For this review, take the finished solid that the model builds, in its own axes (mm). A direction names the side the tool comes from. Round coordinates to 2 decimals unless told otherwise and drop trailing zeros. Write each loop counter-clockwise with the first axis right and the second up, starting at its lowest first coordinate (ties: lowest second). Pieces come first, ordered by that corner, then holes. Notation, with made-up numbers: (83, 59.25) - (108, 59.25) arc R13 ccw to (108, 81.25) - close; hole circle Ø5 at (20.5, 19.25). An arc over 180 degrees is marked (long way). One line per item, written item: value. Start each with the question number.
Q1. Add section D-D on y = -4. Write out the cut boundary in (x, z), and give its area (3 significant figures).
Q2. Tool access review of faces 4 (the face through (-45, 1, 25.4)), 5 (the face through (-88.9, 13, 13)), 6 (the face through (38.1, -13, 38)), 7 (the face through (-64, -38.1, 13)): name each direction out of +Z, -Z, +X, -X, +Y, -Y from which nothing blocks a thin tool from reaching the whole face with its end or side.
Q3. Add section B-B on y = 22. Write out the cut boundary in (x, z), and give its area (3 significant figures).
Q4. Clearance check with flat-ended pins moving along their axes: pin 1 Ø20.5 at (x, z) = (-63.5, 15.5) entering from -Y; pin 2 Ø2 at (y, z) = (-46.5, 12) entering from +X; pin 3 Ø8 at (x, y) = (-69.5, -7.5) entering from +Z. State where each tip first meets the part, or that it passes through.
Q5. Mouldability with a two-part tool opening along Y and no side actions: class faces 1 (the face through (18.78, -35.63, 40.15)), 2 (the face through (21, 63.5, 29)), 3 (the face through (0, 1, 50)) as +Y half, -Y half, draft (parallel to the pull), parting line (faces both ways), or undercut.
Q6. For probe 1 along X at (y, z) = (15, 17); probe 2 along X at (y, z) = (7.5, 63); probe 3 along Z at (x, y) = (-50, -8.5), list the stretches that pass through material, from the lowest coordinate up.
Q7. Add section C-C on x = -49.5. Write out the cut boundary in (y, z), and give its area (3 significant figures).
Q8. Add section A-A on z = 42. Write out the cut boundary in (x, y), and give its area (3 significant figures).
```python
from build123d import *

# Parameters (mm, degrees)
F0_R     = 12.7
F1_DEPTH = 25.4
F2_DEPTH = 76.2
F3_R     = 11.5415853334
F4_DEPTH = 97.028


with BuildPart() as f1:
    # F0 (on Top) → F1 (new body)
    with BuildSketch(Plane.XY):
        Polygon((0, -63.5), (0, 63.5), (-88.9, 63.5), (-88.9, -38.1), (-38.1, -38.1), (-38.1, -63.5), align=None)
        with Locations((-46.3457293808, 16.616050154)):
            Circle(F0_R, mode=Mode.SUBTRACT)
    extrude(amount=F1_DEPTH)

    # F0 (on Top) → F2 (join)
    with BuildSketch(Plane.XY):
        Polygon((88.9, 38.1), (88.9, 63.5), (0, 63.5), (0, -63.5), (38.1, -63.5), (38.1, 38.1), align=None)
    extrude(amount=F2_DEPTH)

    # F3 (on Right) → F4 (cut)
    with BuildSketch(Plane.YZ):
        with Locations((-26.4720246196, 47.1727401018)):
            Circle(F3_R)
    extrude(amount=F4_DEPTH, mode=Mode.SUBTRACT)


solid = f1.part
```
Result set:
1. outline: (-88.9, 0) - (38.1, 0) - (38.1, 76.2) - (0, 76.2) - (0, 25.4) - (-88.9, 25.4) - close
1. area: 5,160 mm^2
2. face 4: +Z, -X, +Y, -Y
2. face 5: +Z, -Z, -X, +Y, -Y
2. face 6: +Z, -Z, +X, -Y
2. face 7: +Z, -Z, -X, -Y
3. outline: (-88.9, 0) - (-57.85, 0) - (-57.85, 25.4) - (-88.9, 25.4) - close; (-34.84, 0) - (38.1, 0) - (38.1, 76.2) - (0, 76.2) - (0, 25.4) - (-34.84, 25.4) - close
3. area: 4,580 mm^2
4. pin 1: stops at y = -38.1
4. pin 2: stops at x = 38.1
4. pin 3: stops at z = 25.4
5. face 1: undercut
5. face 2: +Y half
5. face 3: draft
6. probe 1: x = -88.9 to -58.94, -33.75 to 38.1
6. probe 2: x = 0 to 38.1
6. probe 3: z = 0 to 25.4
7. outline: (-38.1, 0) - (4.31, 0) - (4.31, 25.4) - (-38.1, 25.4) - close; (28.92, 0) - (63.5, 0) - (63.5, 25.4) - (28.92, 25.4) - close
7. area: 1,960 mm^2
8. outline: (0, -63.5) - (38.1, -63.5) - (38.1, -36.79) - (0, -36.79) - close; (0, -16.15) - (38.1, -16.15) - (38.1, 38.1) - (88.9, 38.1) - (88.9, 63.5) - (0, 63.5) - close
8. area: 5,340 mm^2
